```python
from build123d import *

# Parameters (mm, degrees)
F0_W     = 100
F0_H     = 100
F1_DEPTH = 12.7
F2_R     = 5
F3_DEPTH = 25
F2_R_2   = 1
F4_DEPTH = 5


with BuildPart() as f1:
    # F0 (on Top) → F1 (new body)
    with BuildSketch(Plane.XY):
        Rectangle(F0_W, F0_H)
    extrude(amount=F1_DEPTH)

    # F2 (on face) → F3 (cut)
    with BuildSketch(Plane.XY.offset(12.7)):
        Circle(F2_R)
    extrude(amount=-F3_DEPTH, mode=Mode.SUBTRACT)

    # F2 (on face) → F4 (cut)
    with BuildSketch(Plane.XY.offset(12.7)):
        with Locations((-22, 21)):
            Circle(F2_R_2)
        with Locations((22, 21)):
            Circle(F2_R_2)
        with Locations((22, -23)):
            Circle(F2_R_2)
        with Locations((-22, -23)):
            Circle(F2_R_2)
    extrude(amount=-F4_DEPTH, mode=Mode.SUBTRACT)


solid = f1.part
```
Input: part model. Units: mm. Frame: model coordinates. Round coordinates to 2 decimals unless told otherwise and drop trailing zeros. Loops run counter-clockwise (first coordinate to the right, second up) from the corner with the lowest first, then second, coordinate; pieces in that order, holes last. Notation, with made-up numbers: (57, 25.25) -> (80, 25.25) arc R17 ccw to (80, 52.25) -> close; hole circle Ø8 at (-3.5, 66). An arc over 180 degrees is marked (long way). Use one line per item in the form item = value. Start each with the question number.
Item 1: Material intervals for L1, parallel to Y at x = 22, z = 9.9; L2, parallel to Y at x = 0, z = 6.25; L3, parallel to X at y = 1.5, z = 2, sorted ascending. Write a range as from..to.
Item 2: Section query A-A on y = 0. Return the cut outline in (x, z), then the cut area to 3 significant figures.
Item 3: Section query B-B on x = -2.5. Return the cut outline in (y, z), then the cut area to 3 significant figures.
Item 4: Contact query for flat-ended pins moving along their axis: pin 1 Ø13 at (x, y) = (0, 0) entering from -Z; pin 2 Ø1.6 at (x, y) = (-22, 21) entering from +Z. Output: stop coordinate, or through.
Item 5: Mould query, pull axis X, two halves, no side actions, for faces 1 (the face through (50, -1, 6)), 2 (the face through (-1.08, -4.88, 6.44)), 3 (the face through (-1, 12, 0)). Classes: pulls with the +X half, pulls with the -X half, needs draft (parallel to the pull), parting line crosses it, or undercut.
Ans:
q1.L1 = -50..-24, -22..20, 22..50
q1.L2 = -50..-5, 5..50
q1.L3 = -50..-4.77, 4.77..50
q2.outline = (-50, 0) -> (-5, 0) -> (-5, 12.7) -> (-50, 12.7) -> close; (5, 0) -> (50, 0) -> (50, 12.7) -> (5, 12.7) -> close
q2.area = 1,140 mm^2
q3.outline = (-50, 0) -> (-4.33, 0) -> (-4.33, 12.7) -> (-50, 12.7) -> close; (4.33, 0) -> (50, 0) -> (50, 12.7) -> (4.33, 12.7) -> close
q3.area = 1,160 mm^2
q4.pin_1 = 0
q4.pin_2 = 7.7
q5.face_1 = pulls with the +X half
q5.face_2 = undercut
q5.face_3 = needs draft
